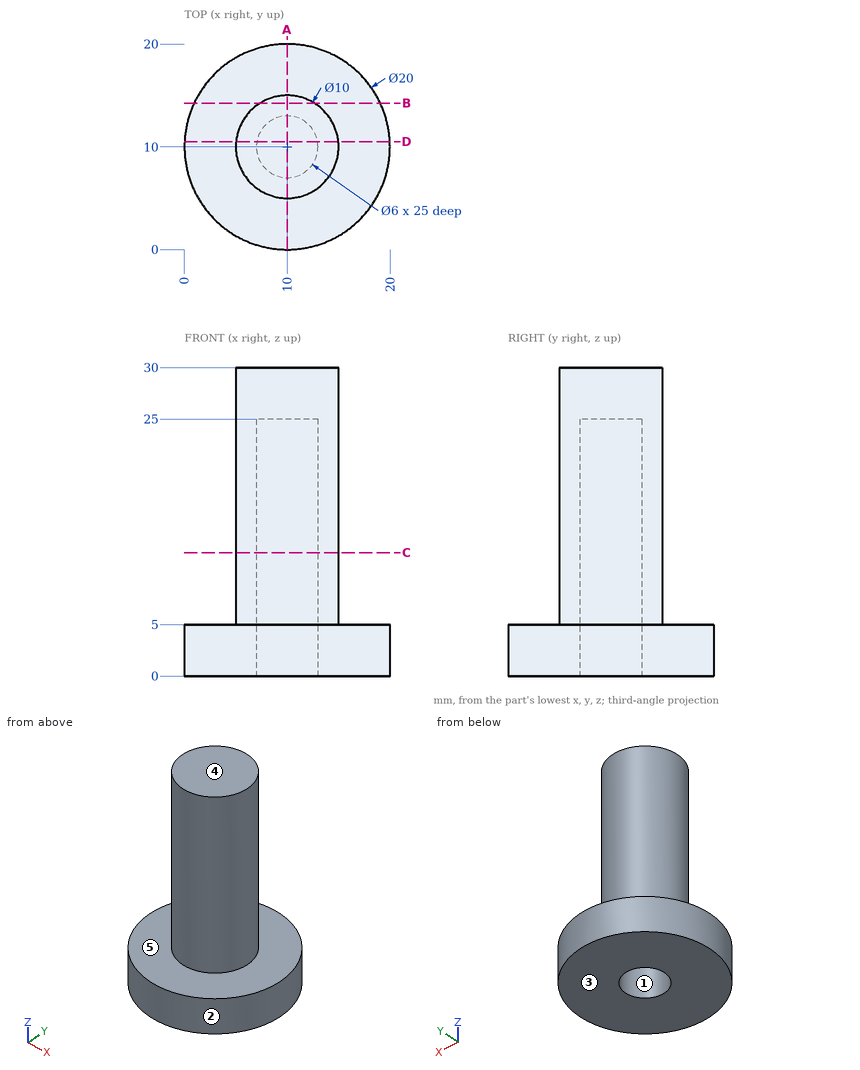
Print and shaded views of the part. All mm, measured from the part's lowest x, y and z. A direction names the side the tool comes from. Coordinates: 2 decimals unless noted, no trailing zeros. Loops run counter-clockwise (first coordinate to the right, second up) from the corner with the lowest first, then second, coordinate; pieces in that order, holes last. Notation, with made-up numbers: (-36, -37) -> (-22, -37) arc R35 ccw to (-22, -1) -> close; hole circle Ø5 at (19.5, 26). An arc over 180 degrees is marked (long way). Use a Markdown table: item, result. Add a question column.
Item 1: Band-saw the part on A-A on x = 10. Write the cut outline in (y, z).
Item 2: Probe probe 1 along Y at (x, z) = (10, 20.25); probe 2 along Z at (x, y) = (3.25, 16.5); probe 3 along Z at (x, y) = (7.75, 11.25). List the from-to ranges inside material, lowest first.
Item 3: Pull direction X, two halves, no side cores. Call the marked faces 1, 2 and 3: +X half, -X half, draft (parallel to the pull), parting line (faces both ways), or undercut.
Item 4: Which spindle directions (+Z, -Z, +X, -X, +Y, -Y) get a long thin tool onto all of the face, cutting with end or side? Do the marked faces 4 and 5. Say none if no direction does.
Item 5: Flat gauge pins, fed straight in: P1, Ø12, axis at y = 4, z = 16, coming from the -X side; P2, Ø1, axis at x = 14, z = 21.5, coming from the -Y side; P3, Ø6, axis at y = 3, z = 5.5, coming from the +X side. Where does each tip first touch, or does it go through?
Item 6: Band-saw the part on D-D on y = 10.5. Write the cut outline in (x, z).
Item 7: Band-saw the part on C-C on z = 12. Write the cut outline in (x, y).
Item 8: Band-saw the part on B-B on y = 14.25. Write the cut outline in (x, z), plus the area to 3 significant figures.
Geometry says:
| question | item | result |
|---|---|---|
| 1 | outline | (0, 0) -> (7, 0) -> (7, 25) -> (13, 25) -> (13, 0) -> (20, 0) -> (20, 5) -> (15, 5) -> (15, 30) -> (5, 30) -> (5, 5) -> (0, 5) -> close |
| 2 | probe 1 | 5 to 7, 13 to 15 |
| 2 | probe 2 | 0 to 5 |
| 2 | probe 3 | 25 to 30 |
| 3 | face 1 | undercut |
| 3 | face 2 | parting line |
| 3 | face 3 | draft |
| 4 | face 4 | +Z, +X, -X, +Y, -Y |
| 4 | face 5 | +Z |
| 5 | P1 | x = 5 |
| 5 | P2 | y = 6.43 |
| 5 | P3 | x = 19.15 |
| 6 | outline | (0.01, 0) -> (7.04, 0) -> (7.04, 25) -> (12.96, 25) -> (12.96, 0) -> (19.99, 0) -> (19.99, 5) -> (14.97, 5) -> (14.97, 30) -> (5.03, 30) -> (5.03, 5) -> (0.01, 5) -> close |
| 7 | outline | circle Ø10 at (10, 10); hole circle Ø6 at (10, 10) |
| 8 | outline | (0.95, 0) -> (19.05, 0) -> (19.05, 5) -> (12.63, 5) -> (12.63, 30) -> (7.37, 30) -> (7.37, 5) -> (0.95, 5) -> close |
| 8 | area | 222 mm² |
